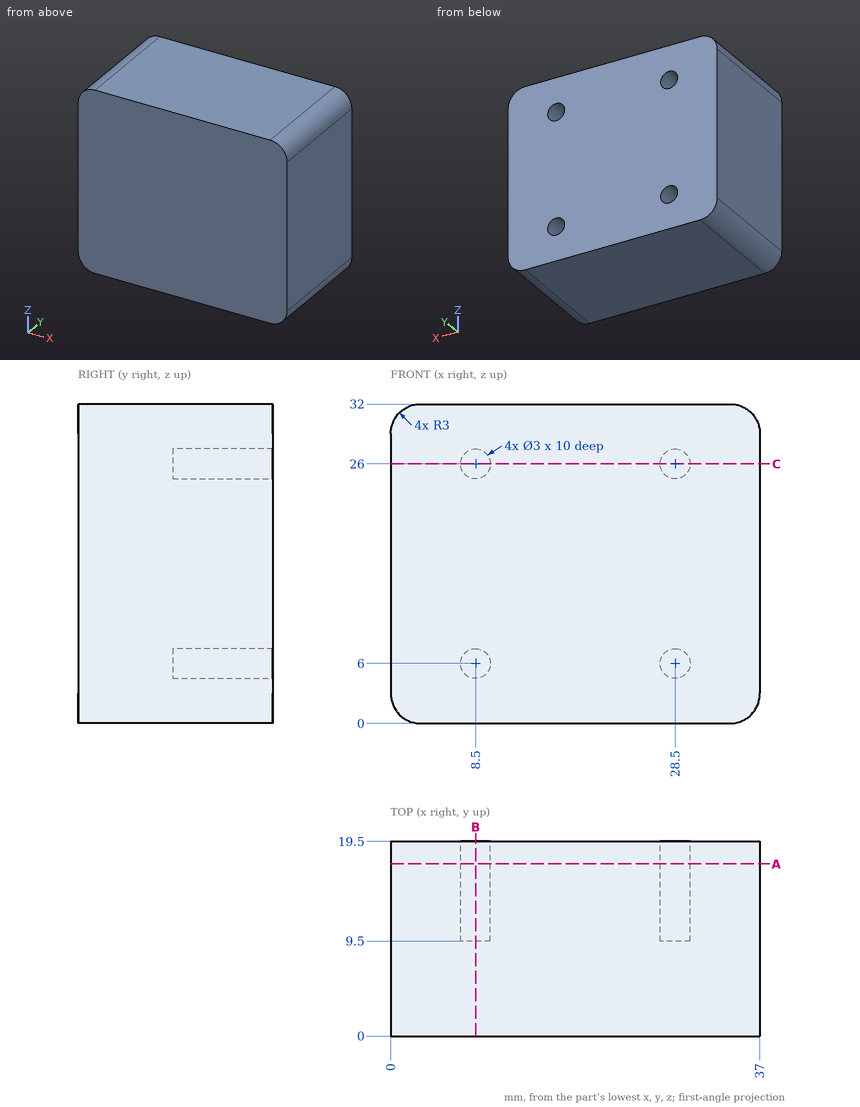
Study the drawing (mm; zero at the part's minimum x, y, z) and answer. Coordinates: 2 decimals unless noted, no trailing zeros. Write each loop counter-clockwise with the first axis right and the second up, starting at its lowest first coordinate (ties: lowest second). Pieces come first, ordered by that corner, then holes. Notation, with made-up numbers: (-14.75, -22.75) - (0.25, -22.75) arc R21 cw to (0.25, -14.75) - close; hole circle Ø1 at (31.5, 60). An arc over 180 degrees is marked (long way). One line per question, with ' | ' between items.
1) Find section A-A, the plane y = 17.25. Determine the outline of the cut face in (x, z).
Checks:
outline: (0, 3) arc R3 ccw to (3, 0) - (34, 0) arc R3 ccw to (37, 3) - (37, 29) arc R3 ccw to (34, 32) - (3, 32) arc R3 ccw to (0, 29) - close; hole circle Ø3 at (8.5, 6); hole circle Ø3 at (8.5, 26); hole circle Ø3 at (28.5, 6); hole circle Ø3 at (28.5, 26)
2) Consider probe 1 along X at (y, z) = (17.5, 26); probe 2 along X at (y, z) = (12.25, 25.5); probe 3 along X at (y, z) = (11.75, 2). Determine where each line is inside the solid, lowest interval first. Write a range as [from, to].
Checks:
probe 1: [0, 7], [10, 27], [30, 37] | probe 2: [0, 7.09], [9.91, 27.09], [29.91, 37] | probe 3: [0.17, 36.83]
3) Find section C-C, the plane z = 26. Determine the outline of the cut face in (x, y).
Checks:
outline: (0, 0) - (37, 0) - (37, 19.5) - (30, 19.5) - (30, 9.5) - (27, 9.5) - (27, 19.5) - (10, 19.5) - (10, 9.5) - (7, 9.5) - (7, 19.5) - (0, 19.5) - close
4) Find section B-B, the plane x = 8.5. Determine the outline of the cut face in (y, z), and give its area (3 significant figures).
Checks:
outline: (0, 0) - (19.5, 0) - (19.5, 4.5) - (9.5, 4.5) - (9.5, 7.5) - (19.5, 7.5) - (19.5, 24.5) - (9.5, 24.5) - (9.5, 27.5) - (19.5, 27.5) - (19.5, 32) - (0, 32) - close | area: 564 mm2
5) Flat-ended cylindrical pins translate along their axes: P1, Ø3.5, axis at x = 28.5, z = 6, coming from the +Y side; P2, Ø0.9, axis at x = 9, z = 6.5, coming from the +Y side. Find the tip coordinate at first contact, or state that the pin passes through.
Checks:
P1: y = 19.5 | P2: y = 9.5
